from build123d import *

# Parameters (mm, degrees)
SKETCH2_R            = 44.45
SKETCH2_R_2          = 38.1
BASE_CYLINDER_DEPTH  = 381
SKETCH3_R            = 56.388
SKETCH3_R_2          = 41.275
AFT_FLANGE_DEPTH     = 17.78
SKETCH4_R            = 56.388
SKETCH4_R_2          = 41.275
FORWARD_FLANGE_DEPTH = 17.78
SKETCH6_R            = 50.0761
SKETCH6_R_2          = 47.0027
O_RING_SLOT_1_DEPTH  = 1.9812
SKETCH7_R            = 50.0761
SKETCH7_R_2          = 47.0027
O_RING_SLOT_2_DEPTH  = 1.9812
FILLET1_R            = 4.7625


with BuildPart() as part:
    # Sketch2 → Base Cylinder (new body)
    with BuildSketch(Plane(origin=(0, 0, 0), x_dir=(1, 0, 0), z_dir=(0, 1, 0))):
        Circle(SKETCH2_R)
        Circle(SKETCH2_R_2, mode=Mode.SUBTRACT)
    extrude(amount=BASE_CYLINDER_DEPTH)

    # Sketch3 → Aft Flange (add)
    with BuildSketch(Plane.XZ):
        Circle(SKETCH3_R)
        Circle(SKETCH3_R_2, mode=Mode.SUBTRACT)
    extrude(amount=-AFT_FLANGE_DEPTH)

    # Sketch4 → Forward Flange (add)
    with BuildSketch(Plane(origin=(0, 381, 0), x_dir=(1, 0, 0), z_dir=(0, 1, 0))):
        Circle(SKETCH4_R)
        Circle(SKETCH4_R_2, mode=Mode.SUBTRACT)
    extrude(amount=-FORWARD_FLANGE_DEPTH)

    # Sketch6 → O-Ring Slot 1 (cut)
    with BuildSketch(Plane.XZ):
        Circle(SKETCH6_R)
        Circle(SKETCH6_R_2, mode=Mode.SUBTRACT)
    extrude(amount=-O_RING_SLOT_1_DEPTH, mode=Mode.SUBTRACT)

    # Sketch7 → O-Ring Slot 2 (cut)
    with BuildSketch(Plane(origin=(0, 381, 0), x_dir=(1, 0, 0), z_dir=(0, 1, 0))):
        Circle(SKETCH7_R)
        Circle(SKETCH7_R_2, mode=Mode.SUBTRACT)
    extrude(amount=-O_RING_SLOT_2_DEPTH, mode=Mode.SUBTRACT)

    # Fillet1
    fillet1_edges = [part.edges().sort_by_distance(p)[0] for p in [
        (-44.45, 363.22, 0),
        (-44.45, 17.78, 0),
    ]]
    fillet(fillet1_edges, radius=FILLET1_R)


solid = part.part
Design review of the part built by this model. Coordinates are the model's own, in mm. A direction names the side the tool comes from. Give positions to 0.01 mm unless a question says otherwise; leave off trailing zeros. Write each loop counter-clockwise with the first axis right and the second up, starting at its lowest first coordinate (ties: lowest second). Pieces come first, ordered by that corner, then holes. Notation, with made-up numbers: M -25.75,21.25 L -14.75,21.25 A15 ccw -14.75,35.25 Z; hole C -5.75,88 d1. An arc over 180 degrees is marked long. Answer as a JSON object with one key per item and string values. Group by question number.
1) We need section A-A (y = 126.5). Give the boundary of the cut face in (x, z).
2) Clearance check with flat-ended pins moving along their axes: pin 1 Ø1 at (y, z) = (290, -28) entering from -X; pin 2 Ø10 at (y, z) = (75, 17) entering from -X; pin 3 Ø4 at (x, y) = (36.5, 117.5) entering from +Z. State where each tip first meets the part, or that it passes through.
3) Mouldability with a two-part tool opening along Z and no side actions: class faces 6 (the face through (-45, 1.981, -15)), 7 (the face through (-44.75, 8.77, -34.31)), 8 (the face through (-30.235, 187.833, 23.183)), 9 (the face through (0, 0, 39)) as released by +Z, released by -Z, zero draft, split by the parting line, or undercut.
4) Tool access review of faces 1 (the face through (-44.75, 372.23, 34.31)), 2 (the face through (25.27, 380.02, -39.63)), 3 (the face through (-10.856, 0.977, -48.885)), 4 (the face through (4, 363.22, -50)), 5 (the face through (0, 381, -39)): name each direction out of +Z, -Z, +X, -X, +Y, -Y from which nothing blocks a thin tool from reaching the whole face with its end or side.
5) For line 1 along Z through (x, y) = (0, 380); line 2 along Y through (x, z) = (-47, 29); line 3 along Z through (x, y) = (0, 268), list the stretches that pass through material, from the lowest coordinate up.
Answer key:
{
 "1": {"outline": "C 0,0 d88.9; hole C 0,0 d76.2"},
 "2": {"pin 1": "stops at x = -34.92", "pin 2": "stops at x = -42.8", "pin 3": "stops at z = 28.03"},
 "3": {"face 6": "undercut", "face 7": "split by the parting line", "face 8": "undercut", "face 9": "zero draft"},
 "4": {"face 1": "+Y, -Y", "face 2": "+Y", "face 3": "-Y", "face 4": "none", "face 5": "+Z, -Z, +X, -X, +Y"},
 "5": {"line 1": "z = -56.39 to -50.08, -47 to -38.1, 38.1 to 47, 50.08 to 56.39", "line 2": "y = 0 to 17.78, 363.22 to 381", "line 3": "z = -44.45 to -38.1, 38.1 to 44.45"}
}
